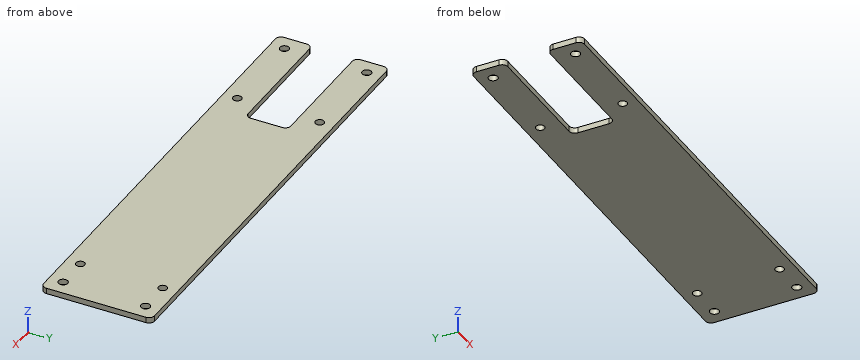
```python
from build123d import *

# Parameters (mm, degrees)
SKETCH_1_W          = 32
SKETCH_1_H          = 39
SKETCH_1_R          = 1.6
SKETCH_1_W_2        = 115
SKETCH_1_R_2        = 1.525
SKETCH_1_W_3        = 12
EXTRUDE_1_DEPTH     = 2
SKETCH_2_W          = 19
SKETCH_2_H          = 15
SKETCH_2_W_2        = 26
CUT_EXTRUDE_1_DEPTH = 10
FILLET_1_R          = 2


with BuildPart() as part:
    # 草图1 → 凸台-拉伸1 (new body)
    # profile 1 of 3: a face of its own
    with BuildSketch(Plane.XY):
        with Locations((-73.5, 0)):
            Rectangle(SKETCH_1_W, SKETCH_1_H)
        with Locations((-84, -14.5)):
            Circle(SKETCH_1_R, mode=Mode.SUBTRACT)
        with Locations((-84, 14.5)):
            Circle(SKETCH_1_R, mode=Mode.SUBTRACT)
    # profile 2 of 3: a face of its own
    with BuildSketch(Plane.XY):
        Rectangle(SKETCH_1_W_2, SKETCH_1_H)
        with Locations((52.5, 14.5)):
            Circle(SKETCH_1_R_2, mode=Mode.SUBTRACT)
        with Locations((52.5, -14.5)):
            Circle(SKETCH_1_R_2, mode=Mode.SUBTRACT)
        with Locations((-52.5, -14.5)):
            Circle(SKETCH_1_R_2, mode=Mode.SUBTRACT)
        with Locations((-52.5, 14.5)):
            Circle(SKETCH_1_R_2, mode=Mode.SUBTRACT)
    # profile 3 of 3: a face of its own
    with BuildSketch(Plane.XY):
        with Locations((63.5, 0)):
            Rectangle(SKETCH_1_W_3, SKETCH_1_H)
        with Locations((64, -14.5)):
            Circle(SKETCH_1_R, mode=Mode.SUBTRACT)
        with Locations((64, 14.5)):
            Circle(SKETCH_1_R, mode=Mode.SUBTRACT)
    extrude(amount=EXTRUDE_1_DEPTH)

    # 草图2 → 切除-拉伸1 (cut)
    with BuildSketch(Plane.XY.offset(2)):
        with Locations((-80, 0)):
            Rectangle(SKETCH_2_W, SKETCH_2_H)
        with Locations((-57.5, 0)):
            Rectangle(SKETCH_2_W_2, SKETCH_2_H)
    extrude(amount=-CUT_EXTRUDE_1_DEPTH, mode=Mode.SUBTRACT)

    # 圆角1
    fillet_1_edges = [part.edges().sort_by_distance(p)[0] for p in [
        (-89.5, 19.5, 1),
        (69.5, 19.5, 1),
        (69.5, -19.5, 1),
        (-89.5, -19.5, 1),
        (-44.5, -7.5, 1),
        (-89.5, -7.5, 1),
        (-89.5, 7.5, 1),
        (-44.5, 7.5, 1),
    ]]
    fillet(fillet_1_edges, radius=FILLET_1_R)


solid = part.part
```
The listing builds one solid part. Answer for the finished solid, in the listing's coordinates (mm). Coordinates: 2 decimals unless noted, no trailing zeros. Write each loop counter-clockwise with the first axis right and the second up, starting at its lowest first coordinate (ties: lowest second). Pieces come first, ordered by that corner, then holes. Notation, with made-up numbers: (-14, 85.5) - (30, 85.5) arc R24 cw to (30, 108.5) - close; hole circle Ø1 at (77.25, 84.5). An arc over 180 degrees is marked (long way). Return JSON: item names as keys, results as strings. Group by question number.
Q1. A flat-ended cylindrical pin translates along its axis: pin 1 Ø1 at (y, z) = (4.5, 1) entering from -X. Find the tip coordinate at first contact, or state that the pin passes through.
Q2. The part is cut by section D-D on x = -52.5. Write down the section's boundary in (y, z) (3 decimals).
Q3. The part is cut by section A-A on x = 52.5. Write down the section's boundary in (y, z) (3 decimals), and give its area (3 significant figures).
Q4. The part is cut by section C-C on y = 14.5. Write down the section's boundary in (x, z) (3 decimals).
Q5. The part is cut by section B-B on z = 1.7. State how many separate pieces and enclosed holes the cut face has, and give its area (3 significant figures).
Q6. Find the intervals of material crossed by line 1 along Y through (x, z) = (52.5, 1.2) (3 decimals); line 2 along Y through (x, z) = (-84, 0.7); line 3 along Y through (x, z) = (64, 0.85), in increasing order. Write a range as [from, to].
Evaluation:
{
 "1": {"pin 1": "stops at x = -44.5"},
 "2": {"outline": "(-19.5, 0) - (-16.025, 0) - (-16.025, 2) - (-19.5, 2) - close; (-12.975, 0) - (-7.5, 0) - (-7.5, 2) - (-12.975, 2) - close; (7.5, 0) - (12.975, 0) - (12.975, 2) - (7.5, 2) - close; (16.025, 0) - (19.5, 0) - (19.5, 2) - (16.025, 2) - close"},
 "3": {"outline": "(-19.5, 0) - (-16.025, 0) - (-16.025, 2) - (-19.5, 2) - close; (-12.975, 0) - (12.975, 0) - (12.975, 2) - (-12.975, 2) - close; (16.025, 0) - (19.5, 0) - (19.5, 2) - (16.025, 2) - close", "area": "65.8 mm2"},
 "4": {"outline": "(-89.5, 0) - (-85.6, 0) - (-85.6, 2) - (-89.5, 2) - close; (-82.4, 0) - (-54.025, 0) - (-54.025, 2) - (-82.4, 2) - close; (-50.975, 0) - (50.975, 0) - (50.975, 2) - (-50.975, 2) - close; (54.025, 0) - (62.4, 0) - (62.4, 2) - (54.025, 2) - close; (65.6, 0) - (69.5, 0) - (69.5, 2) - (65.6, 2) - close"},
 "5": {"separate pieces": "1", "enclosed holes": "8", "area": "5,460 mm2"},
 "6": {"line 1": "y = [-19.5, -16.025], [-12.975, 12.975], [16.025, 19.5]", "line 2": "y = [-19.5, -16.1], [-12.9, -7.5], [7.5, 12.9], [16.1, 19.5]", "line 3": "y = [-19.5, -16.1], [-12.9, 12.9], [16.1, 19.5]"}
}
